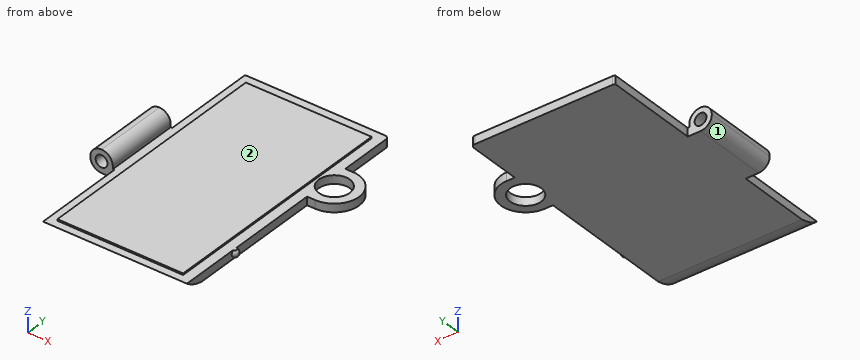
```python
from build123d import *

# Parameters (mm, degrees)
F1_DEPTH  = 3.175
F2_R      = 5
F3_DEPTH  = 3.175
F4_W      = 7.239
F4_H      = 24.13
F5_DEPTH  = 7.239
F6_R      = 1.905
F7_DEPTH  = 25.4
F8_R      = 3.6195
F9_R      = 3.61949
F10_R     = 3.61949
F13_W     = 3.2799700804
F13_H     = 6.7503359169
F14_DEPTH = 0.5
F15_W     = 30.353
F15_H     = 2.675
F16_DEPTH = 0.5
F18_DEPTH = 46.236


# Not quite as in the source:
# - a fillet or chamfer is up to 0.001 mm smaller than in the source, because OpenCascade refuses the exact size


with BuildPart() as f1:
    # F0 (on Top) → F1 (new body)
    with BuildSketch(Plane.XY):
        with BuildLine():
            ThreePointArc((23.368, 41.148), (22.9960256121, 42.0460256121), (22.098, 42.418))
            Line((22.098, 42.418), (-22.098, 42.418))
            ThreePointArc((-22.098, 42.418), (-22.9960256121, 42.0460256121), (-23.368, 41.148))
            Line((-23.368, 41.148), (-23.368, -41.148))
            ThreePointArc((-23.368, -41.148), (-22.9960256121, -42.0460256121), (-22.098, -42.418))
            Line((-22.098, -42.418), (22.098, -42.418))
            ThreePointArc((22.098, -42.418), (22.9960256121, -42.0460256121), (23.368, -41.148))
            Line((23.368, -41.148), (23.368, 8.2812636))
            Line((23.368, 8.2812636), (23.368, 24.2070636))
            Line((23.368, 24.2070636), (23.368, 41.148))
        make_face()
        with BuildLine():
            Line((25.980898, 24.2070636), (23.368, 24.2070636))
            Line((23.368, 24.2070636), (23.368, 8.2812636))
            Line((23.368, 8.2812636), (25.980898, 8.2812636))
            ThreePointArc((25.980898, 8.2812636), (33.943798, 16.2441636), (25.980898, 24.2070636))
        make_face()
    extrude(amount=F1_DEPTH)

    # F2 (on face) → F3 (cut)
    with BuildSketch(Plane.XY.offset(3.175)):
        with Locations((25.980898, 16.2441636)):
            Circle(F2_R)
    extrude(amount=-F3_DEPTH, mode=Mode.SUBTRACT)

    # F4 (on face) → F5 (join)
    with BuildSketch(Plane(origin=(0, 0, 0), x_dir=(1, 0, 0), z_dir=(0, 0, -1))):
        with Locations((-26.9875, 0)):
            Rectangle(F4_W, F4_H)
    extrude(amount=-F5_DEPTH)

    # F6 (on face) → F7 (cut)
    with BuildSketch(Plane.XZ.offset(12.065)):
        with Locations((-26.9875, 3.6195)):
            Circle(F6_R)
    extrude(amount=-F7_DEPTH, mode=Mode.SUBTRACT)

    # F8
    f8_edges = [f1.edges().sort_by_distance(p)[0] for p in [
        (-30.607, 0, 7.239),
    ]]
    fillet(f8_edges, radius=F8_R)

    # F9 (radius 3.6195 in the source; OpenCascade refuses exactly that, so slightly less here)
    f9_edges = [f1.edges().sort_by_distance(p)[0] for p in [
        (-23.368, 0, 7.239),
    ]]
    fillet(f9_edges, radius=F9_R)

    # F10 (radius 3.6195 in the source; OpenCascade refuses exactly that, so slightly less here)
    f10_edges = [f1.edges().sort_by_distance(p)[0] for p in [
        (-30.607, 0, 0),
    ]]
    fillet(f10_edges, radius=F10_R)

    # F11 (on face) → F12 (revolve)
    with BuildSketch(Plane.YZ.offset(23.368)):
        with BuildLine():
            Line((-21.8558364, 2.8575), (-21.8558364, 0.3175))
            ThreePointArc((-21.8558364, 0.3175), (-20.5858364, 1.5875), (-21.8558364, 2.8575))
        make_face()
    revolve(axis=Axis((23.368, -21.8558364, 1.4411548618), (0, 0, 1)))

    # F13 (on face) → F14 (cut)
    with BuildSketch(Plane.XY.offset(3.175)):
        with BuildLine():
            Line((-23.368, -12.065), (-23.368, -42.418))
            Line((-23.368, -42.418), (23.368, -42.418))
            Line((23.368, -42.418), (23.368, -25.3541376442))
            Line((23.368, -25.3541376442), (23.368, -18.6038017273))
            Line((23.368, -18.6038017273), (23.368, 8.2812636))
            Line((23.368, 8.2812636), (25.980898, 8.2812636))
            ThreePointArc((25.980898, 8.2812636), (33.943798, 16.2441636), (25.980898, 24.2070636))
            Line((25.980898, 24.2070636), (23.368, 24.2070636))
            Line((23.368, 24.2070636), (23.368, 42.418))
            Line((23.368, 42.418), (-23.368, 42.418))
            Line((-23.368, 42.418), (-23.368, 12.065))
            Line((-23.368, 12.065), (-23.368, -12.065))
        make_face()
        Polygon((-20.193, 39.243), (20.193, 39.243), (20.193, 22.1750636), (20.193, 10.3132636), (20.193, -39.243), (-20.193, -39.243), (-20.193, -12.065), (-20.193, 12.065), align=None, mode=Mode.SUBTRACT)
        with Locations((25.0079850402, -21.9789696857)):
            Rectangle(F13_W, F13_H)
    extrude(amount=-F14_DEPTH, mode=Mode.SUBTRACT)

    # F15 (on face) → F16 (cut)
    with BuildSketch(Plane(origin=(-23.368, 0, 0), x_dir=(0, -1, 0), z_dir=(-1, 0, 0))):
        with Locations((-27.2415, 1.3375)):
            Rectangle(F15_W, F15_H)
        with Locations((27.2415, 1.3375)):
            Rectangle(F15_W, F15_H)
    extrude(amount=-F16_DEPTH, mode=Mode.SUBTRACT)

    # F17 (on face) → F18 (cut, through all)
    with BuildSketch(Plane(origin=(-22.868, 0, 0), x_dir=(0, -1, 0), z_dir=(-1, 0, 0))):
        with BuildLine():
            ThreePointArc((44.0055, 4.9726288032), (40.2838486613, 1.63965752), (35.5646422155, 0))
            Line((35.5646422155, 0), (44.0055, 0))
            Line((44.0055, 0), (44.0055, 4.9726288032))
        make_face()
    extrude(amount=-F18_DEPTH, mode=Mode.SUBTRACT)


solid = f1.part
```
The listing builds one solid part. Answer for the finished solid, in the listing's coordinates (mm). Face numbers are marked on the shaded views. A direction names the side the tool comes from. Give positions to 0.01 mm unless a question says otherwise; leave off trailing zeros. Loops run counter-clockwise (first coordinate to the right, second up) from the corner with the lowest first, then second, coordinate; pieces in that order, holes last. Notation, with made-up numbers: (75.5, 19) - (82.5, 19) arc R14 ccw to (82.5, 46) - close; hole circle Ø2 at (75.5, 44.5). An arc over 180 degrees is marked (long way). Answer as CSV lines item,"result". Start each with the question number.
Item 1: Each of these flat-tipped pins is pushed along its axis until it touches: pin 1 (1 mm diameter, centred on y = 25.5, z = 2.5, fed in from +X); pin 2 (2 mm diameter, centred on x = -23.5, z = 2.5, fed in from +Y); pin 3 (12 mm diameter, centred on x = 16, y = 14.5, fed in from +Z) (3 decimals); pin 4 (9 mm diameter, centred on x = 25.98, y = 16.24, fed in from -Z). Where does it stop, or does it pass through?
Item 2: A cutting plane is placed at B-B on x = 29. Determine the outline of the cut face in (y, z) (3 decimals).
Item 3: A cutting plane is placed at D-D on x = 14. Determine the outline of the cut face in (y, z) (3 decimals).
Item 4: A cutting plane is placed at C-C on y = 15. Determine the outline of the cut face in (x, z) (3 decimals), then the cut area to 3 significant figures.
Item 5: Find the intervals of material crossed by line 1 (X direction, y = 12, z = 2.25); line 2 (Z direction, x = 3.5, y = 37) (3 decimals); line 3 (Y direction, x = -24, z = 3.75) (3 decimals), in increasing order. Write a range as from..to.
Item 6: For the marked faces 1 and 2, determine the directions among +Z, -Z, +X, -X, +Y, -Y from which every point of the face is accessible in a straight line to the end or side of a thin tool.
Found:
1,pin 1,"stops at x = 23.37"
1,pin 2,"stops at y = 42.35"
1,pin 3,"stops at z = 3.175"
1,pin 4,"passes through"
2,outline,"(8.876, 0) - (12.259, 0) - (12.259, 2.675) - (8.876, 2.675) - close; (20.23, 0) - (23.613, 0) - (23.613, 2.675) - (20.23, 2.675) - close"
3,outline,"(-41.784, 2.675) arc R12.7 ccw to (-35.565, 0) - (42.418, 0) - (42.418, 2.675) - (39.243, 2.675) - (39.243, 3.175) - (-39.243, 3.175) - (-39.243, 2.675) - close"
4,outline,"(-22.868, 0) - (21.138, 0) - (21.138, 2.675) - (20.193, 2.675) - (20.193, 3.175) - (-20.193, 3.175) - (-20.193, 2.675) - (-22.868, 2.675) - close; (30.824, 0) - (33.846, 0) - (33.846, 2.675) - (30.824, 2.675) - close"
4,area,"146 mm^2"
5,line 1,"x = -30.34..-28.31, -25.66..23.34, 28.62..32.72"
5,line 2,"z = 0..3.175"
5,line 3,"y = -12.065..12.065"
6,face 1,"-Z, -X, +Y, -Y"
6,face 2,"+Z, +X, +Y, -Y"
